For this review, take the finished solid that the model builds, in its own axes (mm). A direction names the side the tool comes from. Give positions to 0.01 mm unless a question says otherwise; leave off trailing zeros. Loops run counter-clockwise (first coordinate to the right, second up) from the corner with the lowest first, then second, coordinate; pieces in that order, holes last.
```python
from build123d import *

# Parameters (mm, degrees)
SKETCH_W        = 58.5
SKETCH_H        = 55
PAD004_DEPTH    = 5
SKETCH005_W     = 43
SKETCH005_H     = 24.5
POCKET_DEPTH    = 5
CHAMFER_SIZE    = 2
SKETCH006_R     = 2
POCKET001_DEPTH = 2.5
SKETCH007_R     = 1.05
POCKET002_DEPTH = 5
SKETCH008_W     = 35
SKETCH008_H     = 9.5
POCKET003_DEPTH = 1
FILLET002_R     = 1


with BuildPart() as part:
    # Sketch → Pad004 (new body)
    with BuildSketch(Plane.XZ):
        Rectangle(SKETCH_W, SKETCH_H)
    extrude(amount=PAD004_DEPTH)

    # Sketch005 (on Face6 of Pad004) → Pocket (cut)
    with BuildSketch(Plane.XZ.offset(5)):
        with Locations((0, 8.25)):
            Rectangle(SKETCH005_W, SKETCH005_H)
    extrude(amount=-POCKET_DEPTH, mode=Mode.SUBTRACT)

    # Chamfer
    chamfer_edges = [part.edges().sort_by_distance(p)[0] for p in [
        (-21.5, -5, 8.25),
        (0, -5, 20.5),
        (0, -5, -4),
        (21.5, -5, 8.25),
    ]]
    chamfer(chamfer_edges, length=CHAMFER_SIZE)

    # Sketch006 (on Face1 of Chamfer) → Pocket001 (cut)
    with BuildSketch(Plane.XZ.offset(5)):
        with Locations((-25.75, 24)):
            Circle(SKETCH006_R)
        with Locations((25.75, 24)):
            Circle(SKETCH006_R)
        with Locations((-25.75, -24)):
            Circle(SKETCH006_R)
        with Locations((25.75, -24)):
            Circle(SKETCH006_R)
    extrude(amount=-POCKET001_DEPTH, mode=Mode.SUBTRACT)

    # Sketch007 (on Face16 of Pocket001) → Pocket002 (cut)
    with BuildSketch(Plane.XZ.offset(2.5)):
        with Locations((-25.75, 24)):
            Circle(SKETCH007_R)
        with Locations((25.75, 24)):
            Circle(SKETCH007_R)
        with Locations((25.75, -24)):
            Circle(SKETCH007_R)
        with Locations((-25.75, -24)):
            Circle(SKETCH007_R)
    extrude(amount=-POCKET002_DEPTH, mode=Mode.SUBTRACT)

    # Sketch008 (on Face1 of Pocket002) → Pocket003 (cut)
    with BuildSketch(Plane.XZ.offset(5)):
        with Locations((0, -15.25)):
            Rectangle(SKETCH008_W, SKETCH008_H)
    extrude(amount=-POCKET003_DEPTH, mode=Mode.SUBTRACT)

    # Fillet002
    fillet002_edges = [part.edges().sort_by_distance(p)[0] for p in [
        (29.25, -2.5, 27.5),
        (-29.25, -2.5, 27.5),
        (29.25, -2.5, -27.5),
        (-29.25, -2.5, -27.5),
    ]]
    fillet(fillet002_edges, radius=FILLET002_R)


solid = part.part
```
Item 1: Take a section at B-B on z = -24. Give the boundary of the cut face in (x, y), and give its area (3 significant figures).
Answer:
outline: (-29.25, -5) - (-27.75, -5) - (-27.75, -2.5) - (-26.8, -2.5) - (-26.8, 0) - (-29.25, 0) - close; (-24.7, -2.5) - (-23.75, -2.5) - (-23.75, -5) - (23.75, -5) - (23.75, -2.5) - (24.7, -2.5) - (24.7, 0) - (-24.7, 0) - close; (26.8, -2.5) - (27.75, -2.5) - (27.75, -5) - (29.25, -5) - (29.25, 0) - (26.8, 0) - close
area: 262 mm2
Item 2: Take a section at D-D on x = 14. Give the boundary of the cut face in (y, z), and give its area (3 significant figures).
Answer:
outline: (-5, -27.5) - (0, -27.5) - (0, -4) - (-3, -4) - (-5, -6) - (-5, -10.5) - (-4, -10.5) - (-4, -20) - (-5, -20) - close; (-5, 22.5) - (-3, 20.5) - (0, 20.5) - (0, 27.5) - (-5, 27.5) - close
area: 139 mm2
Item 3: Take a section at C-C on y = -0.8. Give the boundary of the cut face in (x, z).
Answer:
outline: (-29.25, -26.5) arc R1 ccw to (-28.25, -27.5) - (28.25, -27.5) arc R1 ccw to (29.25, -26.5) - (29.25, 26.5) arc R1 ccw to (28.25, 27.5) - (-28.25, 27.5) arc R1 ccw to (-29.25, 26.5) - close; hole circle Ø2.1 at (-25.75, -24); hole circle Ø2.1 at (-25.75, 24); hole (-21.5, -4) - (21.5, -4) - (21.5, 20.5) - (-21.5, 20.5) - close; hole circle Ø2.1 at (25.75, -24); hole circle Ø2.1 at (25.75, 24)
Item 4: Clearance check with flat-ended pins moving along their axes: pin 1 Ø3.5 at (x, z) = (25.75, -24) entering from -Y; pin 2 Ø3 at (x, z) = (-26.5, -23.5) entering from -Y; pin 3 Ø2 at (x, z) = (-12, -17) entering from -Y. State where each tip first meets the part, or that it passes through.
Answer:
pin 1: stops at y = -2.5
pin 2: stops at y = -5
pin 3: stops at y = -4
Item 5: Take a section at A-A on x = -25.75. Give the boundary of the cut face in (y, z).
Answer:
outline: (-5, -27.5) - (0, -27.5) - (0, -25.05) - (-2.5, -25.05) - (-2.5, -26) - (-5, -26) - close; (-5, -22) - (-2.5, -22) - (-2.5, -22.95) - (0, -22.95) - (0, 22.95) - (-2.5, 22.95) - (-2.5, 22) - (-5, 22) - close; (-5, 26) - (-2.5, 26) - (-2.5, 25.05) - (0, 25.05) - (0, 27.5) - (-5, 27.5) - close
Item 6: The part is to be moulded in two halves that separate along X. For faces 1 (the cylindrical face through (-27.337, -3.768, 22.783)), 2 (the flat face through (19, -5, -12)), say which applies: released by +X, released by -X, zero draft, split by the parting line, or undercut.
Answer:
face 1: undercut
face 2: zero draft
Item 7: For L1, parallel to Z at x = -25.75, y = -0.95; L2, parallel to Z at x = -25.75, y = -3.4; L3, parallel to X at y = -2.25, z = 2.5, list the stretches that pass through material, from the lowest coordinate up.
Answer:
L1: z = -27.5 to -25.05, -22.95 to 22.95, 25.05 to 27.5
L2: z = -27.5 to -26, -22 to 22, 26 to 27.5
L3: x = -29.25 to -21.5, 21.5 to 29.25
Item 8: Tool access review of faces 3 (the flat face through (0, -2, -27.5)), 4 (the flat face through (-21.5, -2, 8)), 5 (the flat face through (0, -4, -5)): name each direction out of +Z, -Z, +X, -X, +Y, -Y from which nothing blocks a thin tool from reaching the whole face with its end or side.
Answer:
face 3: -Z, +X, -X, +Y, -Y
face 4: +Y, -Y
face 5: -Y
